```python
from build123d import *

# Parameters (mm, degrees)
SKETCH1_W           = 18.8
SKETCH1_H           = 22.5
BOSS_EXTRUDE1_DEPTH = 37
BOSS_EXTRUDE2_DEPTH = 11
FILLET1_R           = 5
SKETCH3_R           = 1.5
CUT_EXTRUDE1_DEPTH  = 19.8
SKETCH4_W           = 2.5
SKETCH4_H           = 5
BOSS_EXTRUDE3_DEPTH = 5
FILLET2_R           = 0.5
SKETCH5_R           = 1.5
CUT_EXTRUDE2_DEPTH  = 5
SKETCH6_R           = 2.8
CUT_EXTRUDE3_DEPTH  = 19.8
CUT_EXTRUDE4_DEPTH  = 11
SKETCH8_R           = 3
CUT_EXTRUDE5_DEPTH  = 2


with BuildPart() as part:
    # Sketch1 → Boss-Extrude1 (new body)
    with BuildSketch(Plane.XY):
        Rectangle(SKETCH1_W, SKETCH1_H)
    extrude(amount=BOSS_EXTRUDE1_DEPTH)

    # Sketch2 → Boss-Extrude2 (add)
    with BuildSketch(Plane(origin=(0, 0, 0), x_dir=(-1, 0, 0), z_dir=(0, 0, -1))):
        with BuildLine():
            Line((9.4, 6.025985397), (9.4, -6.025985397))
            ThreePointArc((9.4, -6.025985397), (-0.026782234, -11.165651916), (-9.428799853, -5.980822129))
            Line((-9.428799853, -5.980822129), (-9.428799853, 5.980822129))
            ThreePointArc((-9.428799853, 5.980822129), (-0.026782234, 11.165651916), (9.4, 6.025985397))
        make_face()
    extrude(amount=BOSS_EXTRUDE2_DEPTH)

    # Fillet1
    fillet1_edges = [part.edges().sort_by_distance(p)[0] for p in [
        (0, 11.25, 37),
        (0, -11.25, 37),
    ]]
    fillet(fillet1_edges, radius=FILLET1_R)

    # Sketch3 → Cut-Extrude1 (cut, through all)
    with BuildSketch(Plane(origin=(9.4, 0, 0), x_dir=(0, 0, -1), z_dir=(1, 0, 0))):
        with Locations((-5.25, 8.65)):
            Circle(SKETCH3_R)
        with Locations((-5.25, -8.65)):
            Circle(SKETCH3_R)
    extrude(amount=-CUT_EXTRUDE1_DEPTH, mode=Mode.SUBTRACT)

    # Sketch4 → Boss-Extrude3 (add)
    with BuildSketch(Plane.XY.offset(37)):
        Rectangle(SKETCH4_W, SKETCH4_H)
    extrude(amount=BOSS_EXTRUDE3_DEPTH)

    # Fillet2
    fillet2_edges = [part.edges().sort_by_distance(p)[0] for p in [
        (-9.4, 0, 37),
        (9.4, 0, 37),
        (9.4, 11.25, 16),
        (9.4, -11.25, 16),
        (9.4, 9.785533906, 35.535533906),
        (9.4, -9.785533906, 35.535533906),
        (-9.4, -11.25, 16),
        (-9.4, 11.25, 16),
        (-9.4, 9.785533906, 35.535533906),
        (-9.4, -9.785533906, 35.535533906),
        (0, -2.5, 42),
        (0, 2.5, 42),
    ]]
    fillet(fillet2_edges, radius=FILLET2_R)

    # Sketch5 → Cut-Extrude2 (cut)
    with BuildSketch(Plane(origin=(1.25, 0, 0), x_dir=(0, 0, -1), z_dir=(1, 0, 0))):
        with Locations((-39.5, 0)):
            Circle(SKETCH5_R)
    extrude(amount=-CUT_EXTRUDE2_DEPTH, mode=Mode.SUBTRACT)

    # Sketch6 → Cut-Extrude3 (cut, through all)
    with BuildSketch(Plane(origin=(9.4, 0, 0), x_dir=(0, 0, -1), z_dir=(1, 0, 0))):
        with Locations((-25.72, 0)):
            Circle(SKETCH6_R)
    extrude(amount=-CUT_EXTRUDE3_DEPTH, mode=Mode.SUBTRACT)

    # Sketch7 → Cut-Extrude4 (cut)
    with BuildSketch(Plane(origin=(0, 0, -11), x_dir=(-1, 0, 0), z_dir=(0, 0, -1))):
        with BuildLine():
            Line((-8.228799853, 5.62153994), (-8.228799853, -5.62153994))
            ThreePointArc((-8.228799853, -5.62153994), (-0.025432798, -9.965651584), (8.2, -5.663466987))
            Line((8.2, -5.663466987), (8.2, 5.663466987))
            ThreePointArc((8.2, 5.663466987), (-0.025432798, 9.965651584), (-8.228799853, 5.62153994))
        make_face()
    extrude(amount=-CUT_EXTRUDE4_DEPTH, mode=Mode.SUBTRACT)

    # Sketch8 → Cut-Extrude5 (cut)
    with BuildSketch(Plane(origin=(0, 0, 0), x_dir=(-1, 0, 0), z_dir=(0, 0, -1))):
        Circle(SKETCH8_R)
    extrude(amount=-CUT_EXTRUDE5_DEPTH, mode=Mode.SUBTRACT)


solid = part.part
```
Work out the finished part from the listing and answer in its coordinate system (mm). A direction names the side the tool comes from. Round coordinates to 2 decimals unless told otherwise and drop trailing zeros. Write each loop counter-clockwise with the first axis right and the second up, starting at its lowest first coordinate (ties: lowest second). Pieces come first, ordered by that corner, then holes. Notation, with made-up numbers: (58.25, -23) - (92.25, -23) arc R12 ccw to (92.25, -3) - close; hole circle Ø7 at (-34.75, -2.5). An arc over 180 degrees is marked (long way). Return JSON: item names as keys, results as strings. Group by question number.
Q1. The part is cut by section D-D on z = -1.5. Write down the section's boundary in (x, y).
Q2. For faces 4 (the cylindrical face through (0.184, 11.164, -5.423)), 5 (the flat face through (0, 2.5, 39)), 6 (the cylindrical face through (-0.11, 9.965, -5.577)), determine the directions among +Z, -Z, +X, -X, +Y, -Y from which every point of the face is accessible in a straight line to the end or side of a thin tool.
Q3. Find the intervals of material crossed by L1, parallel to Y at x = 4.75, z = 5.25; L2, parallel to X at y = -5.25, z = 18.5; L3, parallel to X at y = 0.5, z = -7, in increasing order.
Q4. The part is cut by section B-B on z = 39.5. Write down the section's boundary in (x, y), then the cut area to 3 significant figures.
Q5. The part is cut by section A-A on y = 0. Count the separate pieces of the cut face and the enclosed holes in it, then the cut area to 3 significant figures.
Q6. Each of these flat-tipped pins is pushed along its axis until it touches: pin 1 Ø10 at (y, z) = (4.5, 15.5) entering from +X; pin 2 Ø8 at (x, y) = (-7.5, 3.5) entering from +Z; pin 3 Ø1.8 at (x, y) = (0.5, 1) entering from -Z; pin 4 Ø6 at (x, z) = (5, -1.5) entering from -Y. Where does it stop, or does it pass through?
Q7. The part is cut by section C-C on x = 0. Write down the section's boundary in (y, z).
Q8. The mould has two halves that part along X. Classify faces 1 (the flat face through (9.429, 0, -5)), 2 (the flat face through (0, 0, 2)), 3 (the cylindrical face through (0.12, 9.82, 35.5)): released by +X, released by -X, zero draft, split by the parting line, or undercut.
Solved:
{
 "1": {"outline": "(-9.4, -6.03) arc R11.17 ccw to (9.43, -5.98) - (9.43, 5.98) arc R11.17 ccw to (-9.4, 6.03) - close; hole (-8.2, -5.66) arc R9.97 ccw to (8.23, -5.62) - (8.23, 5.62) arc R9.97 ccw to (-8.2, 5.66) - close"},
 "2": {"face 4": "-Z, +Y", "face 5": "+Z, +X, -X, +Y", "face 6": "-Z"},
 "3": {"L1": "-11.25 to -10.15, -7.15 to 7.15, 10.15 to 11.25", "L2": "-9.4 to 9.4", "L3": "-9.4 to -8.2, 8.23 to 9.43"},
 "4": {"outline": "(-1.25, -2.5) - (1.25, -2.5) - (1.25, -1.5) - (-1.25, -1.5) - close; (-1.25, 1.5) - (1.25, 1.5) - (1.25, 2.5) - (-1.25, 2.5) - close", "area": "5.00 mm²"},
 "5": {"separate pieces": "3", "enclosed holes": "0", "area": "610 mm²"},
 "6": {"pin 1": "x = 9.4", "pin 2": "z = 37", "pin 3": "z = 2", "pin 4": "y = -11.25"},
 "7": {"outline": "(-11.25, 0) - (-11.17, 0) - (-11.17, -11) - (-9.97, -11) - (-9.97, 0) - (-3, 0) - (-3, 2) - (3, 2) - (3, 0) - (9.97, 0) - (9.97, -11) - (11.17, -11) - (11.17, 0) - (11.25, 0) - (11.25, 32) arc R5 ccw to (6.25, 37) - (2.5, 37) - (2.5, 41.5) arc R0.5 ccw to (2, 42) - (-2, 42) arc R0.5 ccw to (-2.5, 41.5) - (-2.5, 37) - (-6.25, 37) arc R5 ccw to (-11.25, 32) - close; hole circle Ø3 at (-8.65, 5.25); hole circle Ø5.6 at (0, 25.72); hole circle Ø3 at (0, 39.5); hole circle Ø3 at (8.65, 5.25)"},
 "8": {"face 1": "released by +X", "face 2": "undercut", "face 3": "zero draft"}
}
